Input: part model. Units: mm. Frame: model coordinates. Round coordinates to 2 decimals unless told otherwise and drop trailing zeros. Loops run counter-clockwise (first coordinate to the right, second up) from the corner with the lowest first, then second, coordinate; pieces in that order, holes last. Notation, with made-up numbers: M -37,-40 L 12,-40 A19 ccw 12,-22 Z; hole C 1.5,76 d5. An arc over 180 degrees is marked long. Use one line per item in the form item = value. Start each with the question number.
Q1. Section query A-A, the plane y = 5. Output: boundary loops of the cut face in (x, z), and give its area (3 significant figures).
Q2. Section query D-D, the plane y = 17. Output: boundary loops of the cut face in (x, z).
Q3. Mould query, pull axis Y, two halves, no side actions, for faces 1 (the flat face through (-86, 2, 0)), 2 (the flat face through (-82, 21.557, 2)), 3 (the cylindrical face through (49.345, -8.205, 2.535)). Classes: pulls with the +Y half, pulls with the -Y half, needs draft (parallel to the pull), parting line crosses it, or undercut.
Q4. Section query B-B, the plane x = -213. Output: boundary loops of the cut face in (y, z), and give its area (3 significant figures).
Q5. Section query C-C, the plane z = 0.9. Output: boundary loops of the cut face in (x, y), and give its area (3 significant figures).
Q6. First-contact query: P1, Ø1, axis at y = 7.5, z = 4, coming from the +X side. Flat tip, straight axial feed; report the tip coordinate or a pass-through.
Q7. Ray query, line 1 along X through (y, z) = (1, 2); line 2 along X through (y, z) = (9.5, 3.3); line 3 along X through (y, z) = (-15.5, 0.95). Return the intervals inside material, ascending.
```python
from build123d import *

# Parameters (mm, degrees)
EXTRUDE1_DEPTH     = 5
SKETCH2_R          = 10
CUT_EXTRUDE1_DEPTH = 6


with BuildPart() as part:
    # Sketch1 → Extrude1 (new body)
    with BuildSketch(Plane.XY):
        with BuildLine():
            Line((51.513050076, 21.557056146), (-218.486949924, 21.557056146))
            ThreePointArc((-218.486949924, 21.557056146), (-238.486949924, 1.557056146), (-218.486949924, -18.442943854))
            Line((-218.486949924, -18.442943854), (51.513050076, -18.442943854))
            ThreePointArc((51.513050076, -18.442943854), (71.513050076, 1.557056146), (51.513050076, 21.557056146))
        make_face()
    extrude(amount=EXTRUDE1_DEPTH)

    # Sketch2 → Cut-Extrude1 (cut, through all)
    with BuildSketch(Plane.XY.offset(5)):
        with Locations((-218.486949924, 1.557056146)):
            Circle(SKETCH2_R)
        with Locations((51.513050076, 1.557056146)):
            Circle(SKETCH2_R)
    extrude(amount=-CUT_EXTRUDE1_DEPTH, mode=Mode.SUBTRACT)


solid = part.part
```
Results found:
q1.outline = M -238.19,0 L -227.88,0 L -227.88,5 L -238.19,5 Z; M -209.1,0 L 42.12,0 L 42.12,5 L -209.1,5 Z; M 60.9,0 L 71.21,0 L 71.21,5 L 60.9,5 Z
q1.area = 1,360 mm²
q2.outline = M -231.2,0 L 64.22,0 L 64.22,5 L -231.2,5 Z
q3.face_1 = needs draft
q3.face_2 = pulls with the +Y half
q3.face_3 = undercut
q4.outline = M -18.44,0 L -6.8,0 L -6.8,5 L -18.44,5 Z; M 9.92,0 L 21.56,0 L 21.56,5 L 9.92,5 Z
q4.area = 116 mm²
q5.outline = M -218.49,-18.44 L 51.51,-18.44 A20 ccw 51.51,21.56 L -218.49,21.56 A20 ccw Z; hole C -218.49,1.56 d20; hole C 51.51,1.56 d20
q5.area = 11,400 mm²
q6.P1 = 70.76
q7.line_1 = -238.48 to -228.47, -208.5 to 41.53, 61.5 to 71.51
q7.line_2 = -236.84 to -224.56, -212.41 to 45.44, 57.59 to 69.87
q7.line_3 = -228.93 to 61.96
